```python
from build123d import *

# Parameters (mm, degrees)
BOSS_EXTRUDE1_DEPTH = 10
SKETCH2_W           = 0.8
SKETCH2_H           = 12
CUT_EXTRUDE1_DEPTH  = 10
SKETCH3_R           = 1.5
BOSS_EXTRUDE2_DEPTH = 3
FILLET1_R           = 1
SKETCH4_R           = 3
CUT_EXTRUDE2_DEPTH  = 1.5
BOSS_EXTRUDE3_START = 1
SKETCH6_R           = 4
SKETCH6_R_2         = 3.05
BOSS_EXTRUDE3_DEPTH = 1


with BuildPart() as part:
    # Sketch1 → Boss-Extrude1 (new, symmetric)
    with BuildSketch(Plane(origin=(0, 0, 0), x_dir=(0, 0, -1), z_dir=(1, 0, 0))):
        with BuildLine():
            Line((-6, 0), (-7.5, 0))
            Line((-7.5, 0), (-7.5, 10.4))
            ThreePointArc((-7.5, 10.4), (-7.207106781, 11.107106781), (-6.5, 11.4))
            Line((-6.5, 11.4), (6.5, 11.4))
            ThreePointArc((6.5, 11.4), (7.207106781, 11.107106781), (7.5, 10.4))
            Line((7.5, 10.4), (7.5, 0))
            Line((7.5, 0), (6, 0))
            Line((6, 0), (6, 7.9))
            ThreePointArc((6, 7.9), (5.414213562, 9.314213562), (4, 9.9))
            Line((4, 9.9), (-4, 9.9))
            ThreePointArc((-4, 9.9), (-5.414213562, 9.314213562), (-6, 7.9))
            Line((-6, 7.9), (-6, 0))
        make_face()
    extrude(amount=BOSS_EXTRUDE1_DEPTH, both=True)

    # Sketch2 → Cut-Extrude1 (cut)
    with BuildSketch(Plane.XZ.offset(-9.9)):
        Polygon((4.9, -6), (4.1, -6), (4.1, 6), (4.9, 6), (11.86883473, 6), (11.86883473, -6), align=None)
        with Locations((1.5, 0)):
            Rectangle(SKETCH2_W, SKETCH2_H)
    extrude(amount=CUT_EXTRUDE1_DEPTH, mode=Mode.SUBTRACT)

    # Sketch3 → Boss-Extrude2 (add)
    # profile 1 of 2: a face of its own
    with BuildSketch(Plane(origin=(0, 0, 0), x_dir=(1, 0, 0), z_dir=(0, 1, 0))):
        with BuildLine():
            Line((-6.133974596, 7.5), (-4.401923789, 10.5))
            ThreePointArc((-4.401923789, 10.5), (-4.102222521, 11.223542865), (-4, 12))
            ThreePointArc((-4, 12), (0, 16), (4, 12))
            ThreePointArc((4, 12), (4.102222521, 11.223542865), (4.401923789, 10.5))
            Line((4.401923789, 10.5), (6.133974596, 7.5))
            Line((6.133974596, 7.5), (-6.133974596, 7.5))
        make_face()
        with Locations(Location((0, 12, 0), (0, 0, 270))):
            Circle(SKETCH3_R, mode=Mode.SUBTRACT)
    # profile 2 of 2: a face of its own
    with BuildSketch(Plane(origin=(0, 0, 0), x_dir=(1, 0, 0), z_dir=(0, 1, 0))):
        with BuildLine():
            Line((6.133974596, -7.5), (4.401923789, -10.5))
            ThreePointArc((4.401923789, -10.5), (4.102222521, -11.223542865), (4, -12))
            ThreePointArc((4, -12), (0, -16), (-4, -12))
            ThreePointArc((-4, -12), (-4.102222521, -11.223542865), (-4.401923789, -10.5))
            Line((-4.401923789, -10.5), (-6.133974596, -7.5))
            Line((-6.133974596, -7.5), (6.133974596, -7.5))
        make_face()
        with Locations(Location((0, -12, 0), (0, 0, 270))):
            Circle(SKETCH3_R, mode=Mode.SUBTRACT)
    extrude(amount=BOSS_EXTRUDE2_DEPTH)

    # Fillet1
    fillet1_edges = [part.edges().sort_by_distance(p)[0] for p in [
        (0, 3, 7.5),
        (6.133974596, 1.5, 7.5),
        (-6.133974596, 1.5, 7.5),
        (0, 3, -7.5),
        (-6.133974596, 1.5, -7.5),
        (6.133974596, 1.5, -7.5),
    ]]
    fillet(fillet1_edges, radius=FILLET1_R)

    # Sketch4 → Cut-Extrude2 (cut)
    with BuildSketch(Plane(origin=(0, 3, 0), x_dir=(1, 0, 0), z_dir=(0, 1, 0))):
        with Locations(Location((0, -12, 0), (0, 0, 270))):
            Circle(SKETCH4_R)
        with Locations(Location((0, 12, 0), (0, 0, 270))):
            Circle(SKETCH4_R)
    extrude(amount=-CUT_EXTRUDE2_DEPTH, mode=Mode.SUBTRACT)

    # Sketch6 → Boss-Extrude3 (add)
    # profile 1 of 2: a face of its own
    with BuildSketch(Plane.XZ.offset(BOSS_EXTRUDE3_START)):
        with Locations(Location((0, 12, 0), (0, 0, 270))):
            Circle(SKETCH6_R)
        with Locations(Location((0, 12, 0), (0, 0, 270))):
            Circle(SKETCH6_R_2, mode=Mode.SUBTRACT)
    # profile 2 of 2: a face of its own
    with BuildSketch(Plane.XZ.offset(BOSS_EXTRUDE3_START)):
        with Locations(Location((0, -12, 0), (0, 0, 270))):
            Circle(SKETCH6_R)
        with Locations(Location((0, -12, 0), (0, 0, 270))):
            Circle(SKETCH6_R_2, mode=Mode.SUBTRACT)
    extrude(amount=-BOSS_EXTRUDE3_DEPTH)


solid = part.part
```
Check sheet for the modelled part. Datum: model origin and axes. Units: mm. A direction names the side the tool comes from. Coordinates: 2 decimals unless noted, no trailing zeros. Order: outer loops, then holes, each group sorted by start corner. A loop starts at its lowest first (then second) coordinate and runs counter-clockwise, first axis right, second up. Notation, with made-up numbers: (-3, 74.25) -> (45, 74.25) arc R27 cw to (45, 92.25) -> close; hole circle Ø6 at (45, 40). An arc over 180 degrees is marked (long way). Write item = value, one per line. Start each with the question number.
1) Cross-section at C-C (z = 11). Enter the section's corners in (x, y).
2) Cross-section at D-D (z = -10). Enter the section's corners in (x, y).
3) Cross-section at B-B (x = 7.5). Enter the section's corners in (y, z).
4) Mould release check, pull along Z, two halves, no side actions. Record for faces 6 (the cylindrical face through (0.14, 11.099, 7.215)), 7 (the flat face through (0, 4, -6)), 8 (the flat face through (-5.134, 1.545, -9.233)), 9 (the flat face through (-3.2, -1, -12)): +Z half, -Z half, draft (parallel to the pull), parting line (faces both ways), or undercut.
5) Cross-section at A-A (y = 4.5). Enter the section's corners in (x, z).
6) Access from +Z, -Z, +X, -X, +Y, -Y to the whole of each face (thin tool, end or side, straight path). Record for faces 1 (the flat face through (0.1, 0, -7.7)), 2 (the flat face through (0, 11.4, 0)), 3 (the flat face through (4.1, 9.4, -5.6)), 4 (the flat face through (-1.3, 1.5, -10.7)), 5 (the cylindrical face through (0.07, 0.74, -13.5)).
7) Material ranges on L1, parallel to Z at x = 0, y = 1.1; L2, parallel to X at y = -0.7, z = -12; L3, parallel to X at y = 1.15, z = 12, recorded low to high.
8) Go/stop test with flat-tipped pins: P1, Ø1, axis at x = -7, y = 0.5, coming from the -Z side; P2, Ø1.6, axis at y = 9, z = 5, coming from the +X side; P3, Ø4, axis at y = 7, z = -3.5, coming from the -X side; P4, Ø8, axis at x = -0.5, z = -13.5, coming from the +Y side. Record where each tip stops, or that it passes through.
Ans:
q1.outline = (-4.17, 0) -> (-3.87, 0) -> (-3.87, -1) -> (-2.88, -1) -> (-2.88, 0) -> (-1.12, 0) -> (-1.12, 1.5) -> (-2.83, 1.5) -> (-2.83, 3) -> (-4.17, 3) -> close; (1.12, 0) -> (2.88, 0) -> (2.88, -1) -> (3.87, -1) -> (3.87, 0) -> (4.17, 0) -> (4.17, 3) -> (2.83, 3) -> (2.83, 1.5) -> (1.12, 1.5) -> close
q2.outline = (-4.69, 0) -> (-3.46, 0) -> (-3.46, -1) -> (-2.3, -1) -> (-2.3, 0) -> (2.3, 0) -> (2.3, -1) -> (3.46, -1) -> (3.46, 0) -> (4.69, 0) -> (4.69, 3) -> (2.24, 3) -> (2.24, 1.5) -> (-2.24, 1.5) -> (-2.24, 3) -> (-4.69, 3) -> close
q3.outline = (0, -7.5) -> (10.4, -7.5) arc R1 ccw to (11.4, -6.5) -> (11.4, 6.5) arc R1 ccw to (10.4, 7.5) -> (0, 7.5) -> (0, 6) -> (9.9, 6) -> (9.9, -6) -> (0, -6) -> close
q4.face_6 = +Z half
q4.face_7 = undercut
q4.face_8 = -Z half
q4.face_9 = draft
q5.outline = (-10, -7.5) -> (10, -7.5) -> (10, -6) -> (-10, -6) -> close; (-10, 6) -> (10, 6) -> (10, 7.5) -> (-10, 7.5) -> close
q6.face_1 = -Y
q6.face_2 = +Z, -Z, +X, -X, +Y
q6.face_3 = +X, -Y
q6.face_4 = +Y
q6.face_5 = +Y, -Y
q7.L1 = -16 to -13.5, -10.5 to -6, 6 to 10.5, 13.5 to 16
q7.L2 = -4 to -3.05, 3.05 to 4
q7.L3 = -4 to -1.5, 1.5 to 4
q8.P1 = -7.52
q8.P2 = 4.1
q8.P3 = through
q8.P4 = 3
